Here's how the part is built. I have some questions about the finished solid (model axes, mm). A direction names the side the tool comes from. Give positions to 0.01 mm unless a question says otherwise; leave off trailing zeros. Loops run counter-clockwise (first coordinate to the right, second up) from the corner with the lowest first, then second, coordinate; pieces in that order, holes last. Notation, with made-up numbers: M 60,43.25 L 80,43.25 A16 cw 80,65.25 Z; hole C 6.25,70.25 d9. An arc over 180 degrees is marked long. Answer as CSV lines item,"result". Start each with the question number.
Item 1: If we mould it in two halves opening along Z, with no side actions, what happens to faces 1 (the flat face through (6, -20, 70)), 2 (the cylindrical face through (-0.63, 8.06, -42.65)), 3 (the cylindrical face through (-29.97, -1.32, 49.72))? For each: released by +Z, released by -Z, zero draft, split by the parting line, or undercut.
Item 2: I want a section at B-B on x = 0. List the corners of the cut face in (y, z) for me.
Item 3: Will these pins go through, and if not, where does the flat tip stop? P1, Ø16, axis at x = -1.5, y = 5, coming from the +Z side; P2, Ø4, axis at x = -27.5, z = 4.5, coming from the +Y side; P3, Ø5, axis at x = 0, z = -37.5, coming from the +Y side; P4, Ø3, axis at x = 31, z = 16.5, coming from the +Y side.
Item 4: For faces 4 (the flat face through (-5, 9, 100)), 5 (the cylindrical face through (-2.17, -9.76, 85.21)), which set-ups out of +Z, -Z, +X, -X, +Y, -Y let a thin tool reach every point of the face, with its end or its side?
Item 5: I want a section at A-A on y = 0. List the corners of the cut face in (x, z) for me.
Item 6: I want a section at C-C on z = 72.5. List the corners of the cut face in (x, y) for me, plus the area to 3 significant figures.
Item 7: If I drill on line 1 along Y through (x, z) = (0, 73); line 2 along X through (y, z) = (26, 39.5); line 3 along Z through (x, y) = (-37, -19), over which ranges is the centre line in solid material (lowest first)? Write a range as from..to.
Item 8: I want a section at D-D on z = 32. List the corners of the cut face in (x, y) for me.
Autodesk Inventor part; units mm, degrees
ref_plane "Work Plane1" through (-45, 0, 0) normal (1, 0, 0) x (0, 1, 0)
ref_plane "Work Plane2" through (-45, 0, 0) normal (1, 0, 0) x (0, 1, 0)
ref_plane "XZ Plane" through (0, 0, 0) normal (0, 1, 0) x (-1, 0, 0)
sketch "Sketch1" plane through (0, 0, 0) normal (0, 0, 1) x (1, 0, 0)
  circle A0 centre (0, 0) radius 45
  dimension "d0" = 90
extrude "Extrusion1" add sketch "Sketch1" along normal blind 30 and the other way blind 60
sketch "Sketch2" plane through (0, 0, 30) normal (0, 0, 1) x (1, 0, 0)
  circle A0 centre (0, 0) radius 45
  circle A1 centre (0, 0) radius 30
  dimension "d3" = 60
extrude "Extrusion2" add sketch "Sketch2" along normal blind 40 contours A1
sketch "Sketch3" plane through (0, 0, 70) normal (0, 0, 1) x (1, 0, 0)
  circle A0 centre (0, 0) radius 30
  circle A1 centre (0, 0) radius 20
  dimension "d6" = 40
extrude "Extrusion3" add sketch "Sketch3" along normal blind 30 contours A1
sketch "Sketch4" plane through (0, 0, 100) normal (0, 0, 1) x (1, 0, 0)
  circle A0 centre (0, 0) radius 10
  dimension "d9" = 20
extrude "Extrusion4" cut sketch "Sketch4" against normal blind 30
ref_plane "Work Plane1" through (-45, 0, 0) normal (1, 0, 0) x (0, 1, 0)
sketch "Sketch5" plane through (-45, 0, 0) normal (1, 0, 0) x (0, 1, 0)
  point P0 (0, 0)
sketch "Sketch6" plane through (0, 0, 0) normal (1, 0, 0) x (0, 1, 0)
  point P0 (0, 0)
  point P1 (45, 0)
  point P2 (-45, 0)
  point P3 (-30, 0)
  point P4 (30, 0)
ref_plane "Work Plane2" through (-45, 0, 0) normal (1, 0, 0) x (0, 1, 0)
sketch "Sketch7" plane through (-45, 0, 0) normal (1, 0, 0) x (0, 1, 0)
  line L0 (-45, -60) -> (45, -60)
  circle A0 centre (0, -30) radius 15
  point P0 (0, 0)
  dimension "d25" = 30
extrude "Extrusion5" cut sketch "Sketch7" along normal through all
sketch "Sketch8" plane through (0, 0, -60) normal (0, 0, -1) x (-1, 0, 0)
  point P0 (0, 0)
properties part number "cad@57"
Result:
1,face 1,"released by +Z"
1,face 2,"undercut"
1,face 3,"zero draft"
2,outline,"M -45,-60 L 45,-60 L 45,30 L 30,30 L 30,70 L 20,70 L 20,100 L 10,100 L 10,70 L -10,70 L -10,100 L -20,100 L -20,70 L -30,70 L -30,30 L -45,30 Z; hole C 0,-30 d30"
3,P1,"z = 100"
3,P2,"y = 37.08"
3,P3,"y = 45"
3,P4,"y = 33.98"
4,face 4,"+Z, +X, -X, +Y, -Y"
4,face 5,"+Z"
5,outline,"M -45,-60 L 45,-60 L 45,-45 L -45,-45 Z; M -45,-15 L 45,-15 L 45,30 L 30,30 L 30,70 L 20,70 L 20,100 L 10,100 L 10,70 L -10,70 L -10,100 L -20,100 L -20,70 L -30,70 L -30,30 L -45,30 Z"
6,outline,"C 0,0 d40; hole C 0,0 d20"
6,area,"942 mm^2"
7,line 1,"-20..-10, 10..20"
7,line 2,"-14.97..14.97"
7,line 3,"-60..30"
8,outline,"C 0,0 d60"
